```python
from build123d import *

# Parameters (mm, degrees)
SKETCH1_W           = 71.12
SKETCH1_H           = 38.1
BOSS_EXTRUDE1_DEPTH = 3.175
CUT_EXTRUDE1_REACH  = 5.175
SKETCH2_R           = 2.5527


with BuildPart() as part:
    # Sketch1 → Boss-Extrude1 (new body)
    with BuildSketch(Plane.XY):
        with Locations((35.56, 19.05)):
            Rectangle(SKETCH1_W, SKETCH1_H)
    extrude(amount=BOSS_EXTRUDE1_DEPTH)

    # Sketch2 → Cut-Extrude1 (cut, up to next)
    with BuildSketch(Plane(origin=(0, 0, 0), x_dir=(-1, 0, 0), z_dir=(0, 0, -1)), mode=Mode.PRIVATE) as cut_extrude1_sk1:
        with Locations((-6.35, 6.35)):
            Circle(SKETCH2_R)
    cut_extrude1_tool1 = extrude(cut_extrude1_sk1.sketch, amount=-CUT_EXTRUDE1_REACH, mode=Mode.PRIVATE) & part.part
    add(cut_extrude1_tool1.solids().sort_by_distance((6.35, 6.35, 0))[0], mode=Mode.SUBTRACT)
    # Sketch2 → Cut-Extrude1 (cut, up to next)
    with BuildSketch(Plane(origin=(0, 0, 0), x_dir=(-1, 0, 0), z_dir=(0, 0, -1)), mode=Mode.PRIVATE) as cut_extrude1_sk2:
        with Locations((-64.77, 6.35)):
            Circle(SKETCH2_R)
    cut_extrude1_tool2 = extrude(cut_extrude1_sk2.sketch, amount=-CUT_EXTRUDE1_REACH, mode=Mode.PRIVATE) & part.part
    add(cut_extrude1_tool2.solids().sort_by_distance((64.77, 6.35, 0))[0], mode=Mode.SUBTRACT)
    # Sketch2 → Cut-Extrude1 (cut, up to next)
    with BuildSketch(Plane(origin=(0, 0, 0), x_dir=(-1, 0, 0), z_dir=(0, 0, -1)), mode=Mode.PRIVATE) as cut_extrude1_sk3:
        with Locations((-64.77, 31.75)):
            Circle(SKETCH2_R)
    cut_extrude1_tool3 = extrude(cut_extrude1_sk3.sketch, amount=-CUT_EXTRUDE1_REACH, mode=Mode.PRIVATE) & part.part
    add(cut_extrude1_tool3.solids().sort_by_distance((64.77, 31.75, 0))[0], mode=Mode.SUBTRACT)
    # Sketch2 → Cut-Extrude1 (cut, up to next)
    with BuildSketch(Plane(origin=(0, 0, 0), x_dir=(-1, 0, 0), z_dir=(0, 0, -1)), mode=Mode.PRIVATE) as cut_extrude1_sk4:
        with Locations((-6.35, 31.75)):
            Circle(SKETCH2_R)
    cut_extrude1_tool4 = extrude(cut_extrude1_sk4.sketch, amount=-CUT_EXTRUDE1_REACH, mode=Mode.PRIVATE) & part.part
    add(cut_extrude1_tool4.solids().sort_by_distance((6.35, 31.75, 0))[0], mode=Mode.SUBTRACT)


solid = part.part
```
Build history of the part. All positions in model axes, mm. Round coordinates to 2 decimals unless told otherwise and drop trailing zeros. Loops run counter-clockwise (first coordinate to the right, second up) from the corner with the lowest first, then second, coordinate; pieces in that order, holes last. Notation, with made-up numbers: M -37,-33.5 L 20,-33.5 A22 cw 20,-12.5 Z; hole C 25,4 d4. An arc over 180 degrees is marked long. Answer as CSV lines item,"result".
1. Two-plate mould, pull along X, no slides. Class faces 1 (the flat face through (71.12, 19, 2)), 2 (the cylindrical face through (5.172, 29.485, 1.565)), 3 (the flat face through (35, 38.1, 2)), 4 (the flat face through (0, 19, 2)): released by +X, released by -X, zero draft, split by the parting line, or undercut.
Resolved:
face 1,"released by +X"
face 2,"undercut"
face 3,"zero draft"
face 4,"released by -X"
2. Cut at C-C on z = 2.3. Write the cut outline in (x, y).
Resolved:
outline,"M 0,0 L 71.12,0 L 71.12,38.1 L 0,38.1 Z; hole C 6.35,6.35 d5.11; hole C 6.35,31.75 d5.11; hole C 64.77,6.35 d5.11; hole C 64.77,31.75 d5.11"
3. Wall check: probe 1 along Y at (x, z) = (6.5, 1); probe 2 along X at (y, z) = (6.5, 1.2); probe 3 along X at (y, z) = (4.5, 3.05). Give the ranges that are in metal, low to high. Write a range as [from, to].
Resolved:
probe 1,"y = [0, 3.8], [8.9, 29.2], [34.3, 38.1]"
probe 2,"x = [0, 3.8], [8.9, 62.22], [67.32, 71.12]"
probe 3,"x = [0, 4.59], [8.11, 63.01], [66.53, 71.12]"
4. Cut at B-B on x = 64.77. Write the cut outline in (y, z) (3 decimals), then the cut area to 3 significant figures.
Resolved:
outline,"M 0,0 L 3.797,0 L 3.797,3.175 L 0,3.175 Z; M 8.903,0 L 29.197,0 L 29.197,3.175 L 8.903,3.175 Z; M 34.303,0 L 38.1,0 L 38.1,3.175 L 34.303,3.175 Z"
area,"88.5 mm²"
5. Cut at A-A on y = 6.35. Write the cut outline in (x, z) (3 decimals).
Resolved:
outline,"M 0,0 L 3.797,0 L 3.797,3.175 L 0,3.175 Z; M 8.903,0 L 62.217,0 L 62.217,3.175 L 8.903,3.175 Z; M 67.323,0 L 71.12,0 L 71.12,3.175 L 67.323,3.175 Z"
